For this review, take the finished solid that the model builds, in its own axes (mm). A direction names the side the tool comes from. Round coordinates to 2 decimals unless told otherwise and drop trailing zeros. Write each loop counter-clockwise with the first axis right and the second up, starting at its lowest first coordinate (ties: lowest second). Pieces come first, ordered by that corner, then holes. Notation, with made-up numbers: M 78,-18.75 L 94,-18.75 A22 ccw 94,2.25 Z; hole C -3,3 d2. An arc over 180 degrees is marked long. Answer in a Markdown table with one row per item.
```python
from build123d import *

# Parameters (mm, degrees)
SKETCH_1_R          = 1.5
SKETCH_1_R_2        = 4.5
SKETCH_1_R_3        = 2
SKETCH_1_R_4        = 5.2
SKETCH_1_W          = 8.4
SKETCH_1_H          = 4.4
EXTRUDE_1_DEPTH     = 4
CUT_EXTRUDE_1_DEPTH = 10


with BuildPart() as part:
    # 草图1 → 凸台-拉伸1 (new body)
    with BuildSketch(Plane.XY):
        with BuildLine():
            Line((-138.972571837, 141.054738201), (21.027428163, 141.054738201))
            Line((21.027428163, 141.054738201), (87.027428163, 75.054738201))
            Line((87.027428163, 75.054738201), (87.027428163, -4.945261799))
            Line((87.027428163, -4.945261799), (32.205877569, -37.034385558))
            ThreePointArc((32.205877569, -37.034385558), (17.739495323, -37.516550842), (9.428458368, -25.666008097))
            Line((9.428458368, -25.666008097), (7.027428163, -4.945261799))
            Line((7.027428163, -4.945261799), (-90.203942848, 92.286109212))
            Line((-90.203942848, 92.286109212), (-138.972571837, 92.286109212))
            Line((-138.972571837, 92.286109212), (-138.972571837, 141.054738201))
        make_face()
        with Locations((-52.972571837, 135.054738201)):
            Circle(SKETCH_1_R, mode=Mode.SUBTRACT)
        with Locations((47.027428163, 15.054738201)):
            Circle(SKETCH_1_R_2, mode=Mode.SUBTRACT)
        with Locations(Location((-22.972571837, 135.054738201, 0), (0, 0, 180))):
            Circle(SKETCH_1_R, mode=Mode.SUBTRACT)
        with Locations((7.027428163, 135.054738201)):
            Circle(SKETCH_1_R, mode=Mode.SUBTRACT)
        with Locations((67.027428163, 15.054738201)):
            Circle(SKETCH_1_R_3, mode=Mode.SUBTRACT)
        with Locations((67.027428163, 55.054738201)):
            Circle(SKETCH_1_R_3, mode=Mode.SUBTRACT)
        with Locations((27.027428163, 55.054738201)):
            Circle(SKETCH_1_R_3, mode=Mode.SUBTRACT)
        with Locations((27.027428163, 15.054738201)):
            Circle(SKETCH_1_R_3, mode=Mode.SUBTRACT)
        with Locations((47.027428163, 35.054738201)):
            Circle(SKETCH_1_R_3, mode=Mode.SUBTRACT)
        with Locations(Location((-112.972571837, 135.054738201, 0), (0, 0, 180))):
            Circle(SKETCH_1_R, mode=Mode.SUBTRACT)
        with Locations((-82.972571837, 135.054738201)):
            Circle(SKETCH_1_R, mode=Mode.SUBTRACT)
        with Locations((24.527428163, -23.916404969)):
            Circle(SKETCH_1_R_4, mode=Mode.SUBTRACT)
        with Locations((49.784787476, 103.812097514)):
            Circle(SKETCH_1_R, mode=Mode.SUBTRACT)
        with Locations(Location((70.997990912, 82.598894078, 0), (0, 0, 180))):
            Circle(SKETCH_1_R, mode=Mode.SUBTRACT)
        with Locations(Location((28.571584041, 125.025300949, 0), (0, 0, 180))):
            Circle(SKETCH_1_R, mode=Mode.SUBTRACT)
        with Locations((-53.337194475, 63.904642213)):
            Circle(SKETCH_1_R, mode=Mode.SUBTRACT)
        with Locations(Location((-32.123991039, 42.691438778, 0), (0, 0, 180))):
            Circle(SKETCH_1_R, mode=Mode.SUBTRACT)
        with Locations(Location((-74.55039791, 85.117845649, 0), (0, 0, 180))):
            Circle(SKETCH_1_R, mode=Mode.SUBTRACT)
        with Locations((-37.972571837, 135.054738201)):
            Rectangle(SKETCH_1_W, SKETCH_1_H, mode=Mode.SUBTRACT)
        with Locations((-7.972571837, 135.054738201)):
            Rectangle(SKETCH_1_W, SKETCH_1_H, mode=Mode.SUBTRACT)
        with Locations((-97.972571837, 135.054738201)):
            Rectangle(SKETCH_1_W, SKETCH_1_H, mode=Mode.SUBTRACT)
        with Locations((-67.972571837, 135.054738201)):
            Rectangle(SKETCH_1_W, SKETCH_1_H, mode=Mode.SUBTRACT)
        Polygon((55.865905794, 94.619709358), (61.805602756, 88.680012396), (64.916872594, 91.791282234), (58.977175632, 97.730979196), align=None, mode=Mode.SUBTRACT)
        Polygon((34.652702359, 115.832912794), (37.763972196, 118.944182631), (43.703669158, 113.004485669), (40.592399321, 109.893215832), align=None, mode=Mode.SUBTRACT)
        Polygon((-47.256076157, 54.712254058), (-41.316379195, 48.772557096), (-38.205109357, 51.883826933), (-44.144806319, 57.823523895), align=None, mode=Mode.SUBTRACT)
        Polygon((-68.469279592, 75.925457494), (-65.358009755, 79.036727331), (-59.418312793, 73.097030369), (-62.52958263, 69.985760532), align=None, mode=Mode.SUBTRACT)
    extrude(amount=EXTRUDE_1_DEPTH)

    # 草图2 → 切除-拉伸1 (cut)
    with BuildSketch(Plane(origin=(0, 0, 0), x_dir=(-1, 0, 0), z_dir=(0, 0, -1))):
        with BuildLine():
            Line((98.792246858, 103.505713788), (110.418981679, 118.616857906))
            ThreePointArc((110.418981679, 118.616857906), (112.113620797, 119.394251765), (113.713072721, 118.436182616))
            Line((113.713072721, 118.436182616), (122.899473042, 103.325038498))
            ThreePointArc((122.899473042, 103.325038498), (122.933741653, 101.305767071), (121.190489151, 100.286109212))
            Line((121.190489151, 100.286109212), (100.377354008, 100.286109212))
            ThreePointArc((100.377354008, 100.286109212), (98.583028348, 101.402709289), (98.792246858, 103.505713788))
        make_face()
        with BuildLine():
            Line((1.540878081, 37.232518875), (-16.180834634, 28.952587901))
            ThreePointArc((-16.180834634, 28.952587901), (-18.101395793, 29.077384984), (-19.027428163, 30.764570074))
            Line((-19.027428163, 30.764570074), (-19.027428163, 42.748534587))
            ThreePointArc((-19.027428163, 42.748534587), (-18.288705306, 44.30068792), (-16.618248194, 44.706230108))
            Line((-16.618248194, 44.706230108), (1.103464521, 41.002196569))
            ThreePointArc((1.103464521, 41.002196569), (2.680954944, 39.275023825), (1.540878081, 37.232518875))
        make_face()
        Polygon((127.198237985, 127.054738201), (130.972571837, 120.84615804), (130.972571837, 127.054738201), align=None)
        with BuildLine():
            Line((73.446278945, 98.44171591), (92.214930542, 122.835133626))
            ThreePointArc((92.214930542, 122.835133626), (92.424149051, 124.938138124), (90.629823391, 126.054738201))
            Line((90.629823391, 126.054738201), (32.011635988, 126.054738201))
            ThreePointArc((32.011635988, 126.054738201), (30.086594754, 124.59715524), (30.967460822, 122.348954445))
            Line((30.967460822, 122.348954445), (70.816996628, 97.955536729))
            ThreePointArc((70.816996628, 97.955536729), (72.224826028, 97.694659457), (73.446278945, 98.44171591))
        make_face()
        with BuildLine():
            Line((36.616706696, 93.462689168), (-43.937662379, 92.068564807))
            ThreePointArc((-43.937662379, 92.068564807), (-45.813338133, 93.286939697), (-45.386484011, 95.482478917))
            Line((-45.386484011, 95.482478917), (-23.33185922, 117.537103709))
            Line((-23.33185922, 117.537103709), (-7.607283327, 124.857355573))
            Line((-7.607283327, 124.857355573), (37.626273792, 97.168173472))
            ThreePointArc((37.626273792, 97.168173472), (38.51176098, 94.936649095), (36.616706696, 93.462689168))
        make_face()
        with BuildLine():
            Line((29.20140553, 52.49677533), (-23.612246698, 63.53541151))
            Line((-23.612246698, 63.53541151), (-34.805439363, 70.547080779))
            ThreePointArc((-34.805439363, 70.547080779), (-35.670630649, 72.777688158), (-33.778316178, 74.241693343))
            Line((-33.778316178, 74.241693343), (47.490069377, 75.64817492))
            ThreePointArc((47.490069377, 75.64817492), (49.365745131, 74.42980003), (48.93889101, 72.23426081))
            Line((48.93889101, 72.23426081), (29.20140553, 52.49677533))
        make_face()
        with BuildLine():
            Line((-59.027428163, 23.054738201), (-48.755350225, 23.054738201))
            ThreePointArc((-48.755350225, 23.054738201), (-47.831470692, 23.672054769), (-48.048243444, 24.761844982))
            Line((-48.048243444, 24.761844982), (-57.320321382, 34.033922921))
            ThreePointArc((-57.320321382, 34.033922921), (-58.410111596, 34.250695672), (-59.027428163, 33.32681614))
            Line((-59.027428163, 33.32681614), (-59.027428163, 23.054738201))
        make_face()
        with BuildLine():
            Line((-35.027428163, 36.782660262), (-35.027428163, 47.054738201))
            Line((-35.027428163, 47.054738201), (-45.299506102, 47.054738201))
            ThreePointArc((-45.299506102, 47.054738201), (-46.223385635, 46.437421633), (-46.006612883, 45.34763142))
            Line((-46.006612883, 45.34763142), (-36.734534945, 36.075553481))
            ThreePointArc((-36.734534945, 36.075553481), (-35.644744731, 35.85878073), (-35.027428163, 36.782660262))
        make_face()
    extrude(amount=-CUT_EXTRUDE_1_DEPTH, mode=Mode.SUBTRACT)


solid = part.part
```
Q1. Take a section at B-B (z = 1.7). State how many separate pieces and enclosed holes the cut face has, then the cut area to 3 significant figures.
Found:
| item | result |
|---|---|
| separate pieces | 1 |
| enclosed holes | 34 |
| area | 17,900 mm² |
Q2. Mouldability with a two-part tool opening along X and no side actions: class faces 3 (the face through (1, 52, 4)), 4 (the face through (-82.7, 110.47, 1.97)), 5 (the face through (7.2, 33.15, 1.97)), 6 (the face through (-40.91, 42.99, 1.97)) as +X half, -X half, draft (parallel to the pull), parting line (faces both ways), or undercut.
Found:
| item | result |
|---|---|
| face 3 | draft |
| face 4 | undercut |
| face 5 | undercut |
| face 6 | -X half |
Q3. For probe 1 along X at (y, z) = (36, 3.65); probe 2 along Y at (x, z) = (26, 0.9); probe 3 along Y at (x, z) = (-53, 3.4), list the stretches that pass through material, from the lowest coordinate up.
Found:
| item | result |
|---|---|
| probe 1 | -33.92 to 1.1, 19.03 to 35.4, 36.65 to 45.26, 48.79 to 87.03 |
| probe 2 | -39.04 to -28.9, -18.93 to 13.34, 16.77 to 53.34, 56.77 to 65.03, 74.38 to 92.38, 114.87 to 136.08 |
| probe 3 | 55.08 to 62.44, 65.37 to 108.86, 126.05 to 133.55, 136.55 to 141.05 |
Q4. Take a section at C-C (y = -13.5). State the section outline as (x, z) points, then the cut area to 3 significant figures.
Found:
| item | result |
|---|---|
| outline | M 8.02,0 L 72.41,0 L 72.41,4 L 8.02,4 Z |
| area | 258 mm² |
Q5. Take a section at A-A (x = -15). State the section outline as (y, z) points.
Found:
| item | result |
|---|---|
| outline | M 17.08,0 L 55.47,0 L 55.47,4 L 17.08,4 Z; M 75.09,0 L 93.09,0 L 93.09,4 L 75.09,4 Z; M 111.02,0 L 141.05,0 L 141.05,4 L 111.02,4 Z |
Q6. Machinability: for faces 1 (the face through (1, 52, 0)), 2 (the face through (15.58, 121.146, 1.972)), which of the approach directions +Z, -Z, +X, -X, +Y, -Y give a long, thin tool a straight path to every point of the face, cutting with its end or side? Answer none if there is none.
Found:
| item | result |
|---|---|
| face 1 | -Z, +X, -X, +Y, -Y |
| face 2 | +Z, -Z |
Q7. Insertion check: P1, Ø10, axis at x = -58.5, y = 50, coming from the -Z side; P2, Ø2, axis at x = -7, z = 3, coming from the -Y side; P3, Ø1.2, axis at x = 41.5, z = 1, coming from the -Y side; P4, Ø2, axis at y = 135, z = 1, coming from the +X side. Each pin has a flat end and moves straight along its axis. Give the tip position at first contact, or say it passes through.
Found:
| item | result |
|---|---|
| P1 | through |
| P2 | y = 8.08 |
| P3 | y = -31.95 |
| P4 | x = 28.08 |
